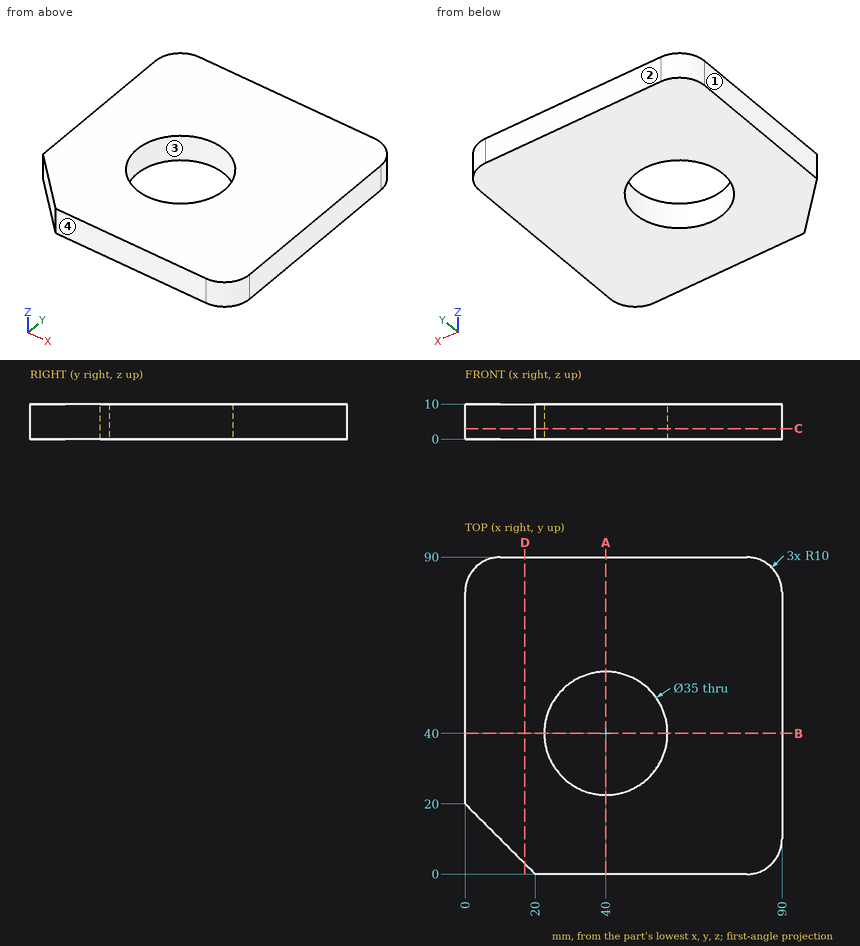
Geometry check sheet. Reference: drawing and pictorial views, mm from the part's lowest x, y, z. Round coordinates to 2 decimals unless told otherwise and drop trailing zeros. Loops run counter-clockwise (first coordinate to the right, second up) from the corner with the lowest first, then second, coordinate; pieces in that order, holes last. Notation, with made-up numbers: (28, -38) - (53, -38) arc R30 cw to (53, -8) - close; hole circle Ø9 at (-2, -3). An arc over 180 degrees is marked (long way). Answer in a Markdown table with one row per item. Add a question column.
Q1. Gauge pin test, flat end, axial feed: pin 1 (21 mm diameter, centred on x = 40, y = 40, fed in from -Z). Record the tip position at first contact, or that the pin passes through.
Q2. Section check C-C on z = 3. Enter the section's corners in (x, y), plus the area to 3 significant figures.
Q3. Section check A-A on x = 40. Enter the section's corners in (y, z), plus the area to 3 significant figures.
Q4. Release check for a two-part mould opening along Y. For the marked faces 1, 2, 3 and 4 record: pulls with the +Y half, pulls with the -Y half, needs draft (parallel to the pull), parting line crosses it, or undercut.
Q5. Material ranges on line 1 (Y direction, x = 40, z = 5.25); line 2 (Y direction, x = 48.5, z = 7.75); line 3 (X direction, y = 45.5, z = 8.5), recorded low to high.
Q6. Section check D-D on x = 17. Enter the section's corners in (y, z), plus the area to 3 significant figures.
Found:
| question | item | result |
|---|---|---|
| 1 | pin 1 | passes through |
| 2 | outline | (0, 20) - (20, 0) - (80, 0) arc R10 ccw to (90, 10) - (90, 80) arc R10 ccw to (80, 90) - (10, 90) arc R10 ccw to (0, 80) - close; hole circle Ø35 at (40, 40) |
| 2 | area | 6,870 mm² |
| 3 | outline | (0, 0) - (22.5, 0) - (22.5, 10) - (0, 10) - close; (57.5, 0) - (90, 0) - (90, 10) - (57.5, 10) - close |
| 3 | area | 550 mm² |
| 4 | face 1 | needs draft |
| 4 | face 2 | pulls with the +Y half |
| 4 | face 3 | undercut |
| 4 | face 4 | pulls with the -Y half |
| 5 | line 1 | y = 0 to 22.5, 57.5 to 90 |
| 5 | line 2 | y = 0 to 24.7, 55.3 to 90 |
| 5 | line 3 | x = 0 to 23.39, 56.61 to 90 |
| 6 | outline | (3, 0) - (90, 0) - (90, 10) - (3, 10) - close |
| 6 | area | 870 mm² |
